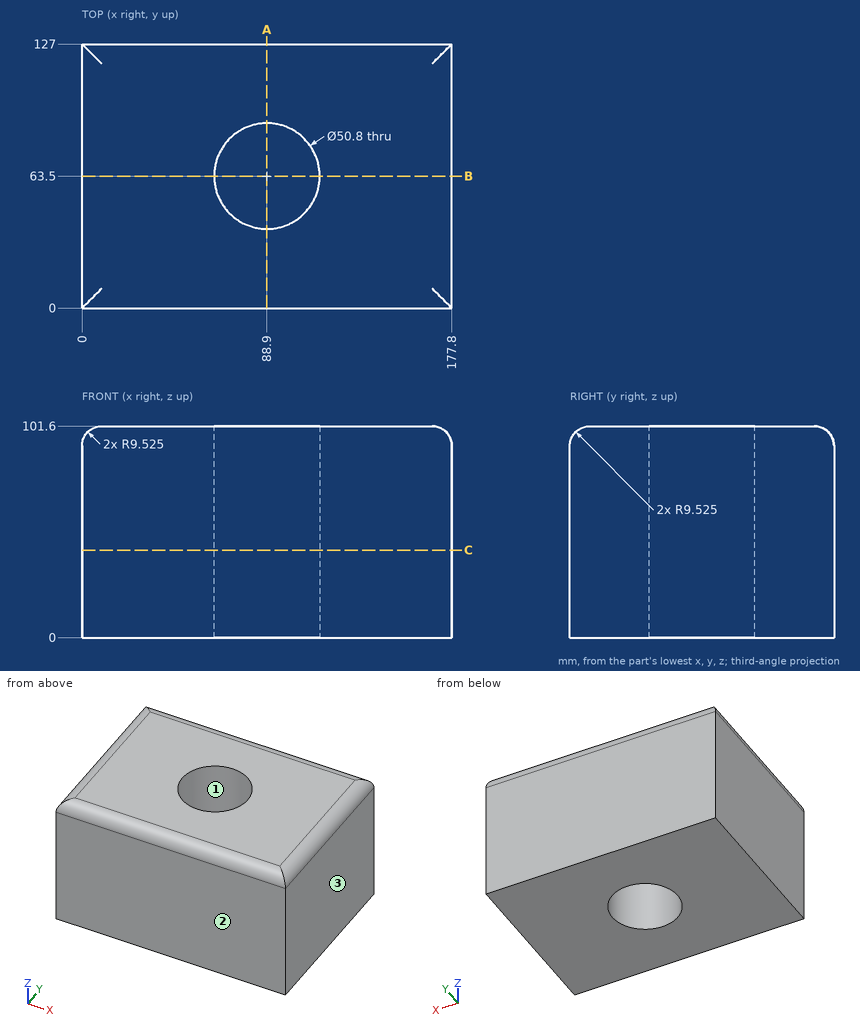
Check sheet for the drawn part. Datum: minimum x, y, z corner. Units: mm. Coordinates: 2 decimals unless noted, no trailing zeros. Write each loop counter-clockwise with the first axis right and the second up, starting at its lowest first coordinate (ties: lowest second). Pieces come first, ordered by that corner, then holes. Notation, with made-up numbers: M -14.75,19 L 16.25,19 A30 cw 16.25,58 Z; hole C 76.5,19 d1. An arc over 180 degrees is marked long. Use a Markdown table: item, result.
Q1. Thickness scan on line 1 (X direction, y = 63, z = 46); line 2 (Y direction, x = 88.9, z = 35.5); line 3 (X direction, y = 22.5, z = 93). Record the ranges inside material, lowest first.
Reply:
| item | result |
|---|---|
| line 1 | x = 0 to 63.5, 114.3 to 177.8 |
| line 2 | y = 0 to 38.1, 88.9 to 127 |
| line 3 | x = 0.05 to 177.75 |
Q2. Sectioned sample at B-B, the plane y = 63.5. Record the boundary of the cut face in (x, z) (3 decimals), plus the area to 3 significant figures.
Reply:
| item | result |
|---|---|
| outline | M 0,0 L 63.5,0 L 63.5,101.6 L 9.525,101.6 A9.525 ccw 0,92.075 Z; M 114.3,0 L 177.8,0 L 177.8,92.075 A9.525 ccw 168.275,101.6 L 114.3,101.6 Z |
| area | 12,900 mm² |
Q3. Sectioned sample at C-C, the plane z = 42. Record the boundary of the cut face in (x, y), plus the area to 3 significant figures.
Reply:
| item | result |
|---|---|
| outline | M 0,0 L 177.8,0 L 177.8,127 L 0,127 Z; hole C 88.9,63.5 d50.8 |
| area | 20,600 mm² |
Q4. Draft check along Y on the marked faces 1, 2 and 3. Enter one of: +Y half, -Y half, draft (parallel to the pull), parting line (faces both ways), or undercut.
Reply:
| item | result |
|---|---|
| face 1 | undercut |
| face 2 | -Y half |
| face 3 | draft |
Q5. Sectioned sample at A-A, the plane x = 88.9. Record the boundary of the cut face in (y, z) (3 decimals).
Reply:
| item | result |
|---|---|
| outline | M 0,0 L 38.1,0 L 38.1,101.6 L 9.525,101.6 A9.525 ccw 0,92.075 Z; M 88.9,0 L 127,0 L 127,92.075 A9.525 ccw 117.475,101.6 L 88.9,101.6 Z |
